```python
from build123d import *

# Parameters (mm, degrees)
SKETCH1_W             = 72.675
SKETCH1_H             = 127
BOSS_EXTRUDE1_DEPTH   = 1.016
SKETCH2_R             = 2.25
CUT_EXTRUDE1_DEPTH    = 2.016
BOSS_EXTRUDE2_DEPTH   = 1.016
F_6_CLEARANCE_HOLE1_D = 3.7973
FILLET1_R             = 6.35


with BuildPart() as part:
    # Sketch1 → Boss-Extrude1 (new body)
    with BuildSketch(Plane(origin=(0, 0, 0), x_dir=(1, 0, 0), z_dir=(0, 1, 0))):
        with Locations((-38.990743482, -0.569490469)):
            Rectangle(SKETCH1_W, SKETCH1_H)
    extrude(amount=BOSS_EXTRUDE1_DEPTH)

    # Sketch2 → Cut-Extrude1 (cut, through all)
    with BuildSketch(Plane.XZ):
        with Locations((-64.740743482, 8.569490469)):
            Circle(SKETCH2_R)
        with Locations((-64.740743482, -7.430509531)):
            Circle(SKETCH2_R)
        with Locations((-13.240743482, -7.430509531)):
            Circle(SKETCH2_R)
        with Locations((-13.240743482, 8.569490469)):
            Circle(SKETCH2_R)
    extrude(amount=-CUT_EXTRUDE1_DEPTH, mode=Mode.SUBTRACT)

    # Sketch3 → Boss-Extrude2 (add)
    with BuildSketch(Plane(origin=(0, 1.016, 0), x_dir=(1, 0, 0), z_dir=(0, 1, 0))):
        with BuildLine():
            Line((-80.265743482, 37.530509531), (-75.328243482, 37.530509531))
            Line((-75.328243482, 37.530509531), (-75.328243482, 24.830509531))
            Line((-75.328243482, 24.830509531), (-80.265743482, 24.830509531))
            ThreePointArc((-80.265743482, 24.830509531), (-86.615743482, 31.180509531), (-80.265743482, 37.530509531))
        make_face()
        with BuildLine():
            Line((2.284256518, 24.830509531), (-2.653243482, 24.830509531))
            Line((-2.653243482, 24.830509531), (-2.653243482, 37.530509531))
            Line((-2.653243482, 37.530509531), (2.284256518, 37.530509531))
            ThreePointArc((2.284256518, 37.530509531), (8.634256518, 31.180509531), (2.284256518, 24.830509531))
        make_face()
        with BuildLine():
            Line((-75.328243482, -38.669490469), (-75.328243482, -25.969490469))
            Line((-75.328243482, -25.969490469), (-80.265743482, -25.969490469))
            ThreePointArc((-80.265743482, -25.969490469), (-86.615743482, -32.319490469), (-80.265743482, -38.669490469))
            Line((-80.265743482, -38.669490469), (-75.328243482, -38.669490469))
        make_face()
        with BuildLine():
            Line((2.284256518, -25.969490469), (-2.653243482, -25.969490469))
            Line((-2.653243482, -25.969490469), (-2.653243482, -38.669490469))
            Line((-2.653243482, -38.669490469), (2.284256518, -38.669490469))
            ThreePointArc((2.284256518, -38.669490469), (8.634256518, -32.319490469), (2.284256518, -25.969490469))
        make_face()
    extrude(amount=-BOSS_EXTRUDE2_DEPTH)

    # #6 Clearance Hole1 (through all)
    with Locations(Plane(origin=(0, 1.016, 0), x_dir=(1, 0, 0), z_dir=(0, 1, 0))):
        with Locations((-80.265743482, 31.180509531), (-80.265743482, -32.319490469), (2.284256518, -32.319490469), (2.284256518, 31.180509531)):
            Hole(F_6_CLEARANCE_HOLE1_D / 2)

    # Fillet1
    fillet1_edges = [part.edges().sort_by_distance(p)[0] for p in [
        (-75.328243482, 0.508, -37.530509531),
        (-75.328243482, 0.508, -24.830509531),
        (-75.328243482, 0.508, 25.969490469),
        (-75.328243482, 0.508, 38.669490469),
        (-2.653243482, 0.508, -24.830509531),
        (-2.653243482, 0.508, -37.530509531),
        (-2.653243482, 0.508, 25.969490469),
        (-2.653243482, 0.508, 38.669490469),
    ]]
    fillet(fillet1_edges, radius=FILLET1_R)


solid = part.part
```
Geometry check sheet. Reference: the model listing, model coordinates, mm. Coordinates: 2 decimals unless noted, no trailing zeros. Order: outer loops, then holes, each group sorted by start corner. A loop starts at its lowest first (then second) coordinate and runs counter-clockwise, first axis right, second up. Notation, with made-up numbers: (-19, 48.5) - (-10, 48.5) arc R20 ccw to (-10, 71.5) - close; hole circle Ø6 at (12.5, -1.75). An arc over 180 degrees is marked (long way). Answer as a JSON object with one key per item and string values. Group by question number.
Item 1: Depth check by flat-ended pin: pin 1 Ø0.5 at (y, z) = (0.5, -57.5) entering from +X. Enter the tip coordinate at first touch or a pass-through.
Item 2: Sectioned sample at C-C, the plane y = 0.75. Give the number of separate pieces and of enclosed holes in the cut face, and give its area (3 significant figures).
Item 3: Sectioned sample at D-D, the plane z = 28. Record the cut outline in (x, y).
Item 4: Sectioned sample at B-B, the plane z = -51.5. Record the cut outline in (x, y).
Item 5: Draft check along X on faces 1 (the face through (-86.614, 0.515, 32.19)), 2 (the face through (-40, 1.016, 0)), 3 (the face through (8.633, 0.515, -31.31)), 4 (the face through (-78.9, 0.5, 31)). Enter one of: +X half, -X half, draft (parallel to the pull), parting line (faces both ways), or undercut.
Item 6: Sectioned sample at A-A, the plane x = -64. Record the cut outline in (y, z), and give its area (3 significant figures).
Item 7: Scan lines: probe 1 along Z at (x, y) = (-14.5, 0.1); probe 2 along Z at (x, y) = (-13, 0.3); probe 3 along Z at (x, y) = (-79, 0.25). Record each from-to range of solid material in increasing order.
Resolved:
{
 "1": {"pin 1": "x = -2.65"},
 "2": {"separate pieces": "1", "enclosed holes": "8", "area": "9,690 mm^2"},
 "3": {"outline": "(-84.92, 0) - (6.94, 0) - (6.94, 1.02) - (-84.92, 1.02) - close"},
 "4": {"outline": "(-75.33, 0) - (-2.65, 0) - (-2.65, 1.02) - (-75.33, 1.02) - close"},
 "5": {"face 1": "-X half", "face 2": "draft", "face 3": "+X half", "face 4": "undercut"},
 "6": {"outline": "(0, -62.93) - (1.02, -62.93) - (1.02, -9.56) - (0, -9.56) - close; (0, -5.31) - (1.02, -5.31) - (1.02, 6.44) - (0, 6.44) - close; (0, 10.69) - (1.02, 10.69) - (1.02, 64.07) - (0, 64.07) - close", "area": "120 mm^2"},
 "7": {"probe 1": "-62.93 to -9.3, -5.57 to 6.7, 10.43 to 64.07", "probe 2": "-62.93 to -9.67, -5.19 to 6.33, 10.81 to 64.07", "probe 3": "-38.04 to -32.6, -29.77 to -24.32, 25.46 to 30.9, 33.73 to 39.18"}
}
